Autodesk Inventor part; units mm, degrees
ref_plane "YZ Plane" through (0, 0, 0) normal (1, 0, 0) x (0, 1, 0)
ref_plane "XZ Plane" through (0, 0, 0) normal (0, 1, 0) x (-1, 0, 0)
ref_plane "XY Plane" through (0, 0, 0) normal (0, 0, 1) x (1, 0, 0)
sketch "Sketch1" plane through (0, 0, 0) normal (0, 1, 0) x (-1, 0, 0)
  circle A0 centre (0, 0) radius 40.5
  circle A1 centre (0, 0) radius 61
  dimension "d0" = 81
  dimension "d1" = 122
extrude "Extrusion1" add sketch "Sketch1" along normal blind 24
sketch "Sketch2" plane through (0, 24, 0) normal (0, 1, 0) x (1, 0, 0)
  circle A0 centre (0, 0) radius 51 construction
  point P0 (-51, 0)
  point P1 (25.5, -44.1673)
  point P2 (25.5, 44.1673)
  dimension "d4" = 102
  dimension "d7" = 360
hole "Hole1" at (-51, 24, 0) at (25.5, 24, 44.1673) at (25.5, 24, -44.1673) direction (0, -1, 0) diameter 5.5 end through all
properties part number "Adapter"
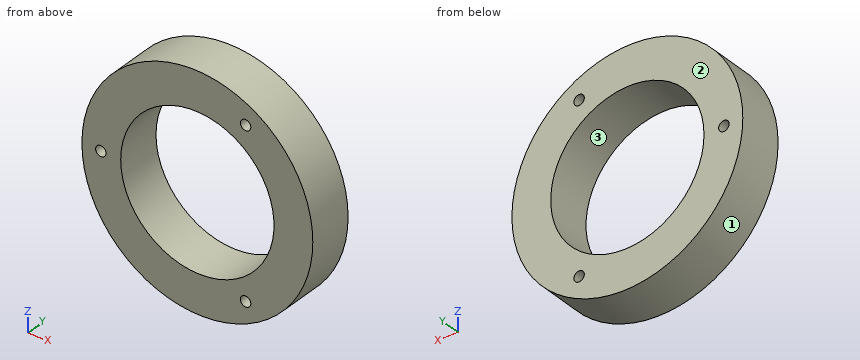
Geometry: final body of the model. Coordinates: model frame, mm. Face numbers are marked on the shaded views. Coordinates: 2 decimals unless noted, no trailing zeros. Order: outer loops, then holes, each group sorted by start corner. A loop starts at its lowest first (then second) coordinate and runs counter-clockwise, first axis right, second up.
(1) Section query D-D (y = 15). Return the cut outline in (x, z), plus the area to 3 significant figures.
(2) Material intervals for probe 1 along Z at (x, y) = (25.5, 7); probe 2 along Z at (x, y) = (27, 16.5); probe 3 along Z at (x, y) = (0, 12.75), sorted ascending.
(3) First-contact query: pin 1 (8 mm diameter, centred on x = -23, y = 6.5, fed in from +Z); pin 2 (8 mm diameter, centred on x = -39, z = -2.5, fed in from +Y); pin 3 (1.5 mm diameter, centred on y = 6, z = -31.5, fed in from -X); pin 4 (1 mm diameter, centred on x = 40.5, y = 12.5, fed in from -Z). Flat tips, straight axial feed; report the tip coordinate or a pass-through.
(4) Draft query along Z for the marked faces 1, 2 and 3. Return one class per face: pulls with the +Z half, pulls with the -Z half, needs draft (parallel to the pull), parting line crosses it, or undercut.
(5) Section query A-A (x = 0). Return the cut outline in (y, z).
(6) Section query B-B (z = 0). Return the cut outline in (x, y).
(7) Section query C-C (z = -23). Return the cut outline in (x, y).
Solution:
1. outline: circle Ø122 at (0, 0); hole circle Ø5.5 at (-51, 0); hole circle Ø81 at (0, 0); hole circle Ø5.5 at (25.5, -44.17); hole circle Ø5.5 at (25.5, 44.17)
1. area: 6,470 mm2
2. probe 1: z = -55.41 to -46.92, -41.42 to -31.46, 31.46 to 41.42, 46.92 to 55.41
2. probe 2: z = -54.7 to -46.47, -41.86 to -30.19, 30.19 to 41.86, 46.47 to 54.7
2. probe 3: z = -61 to -40.5, 40.5 to 61
3. pin 1: stops at z = 57.97
3. pin 2: stops at y = 24
3. pin 3: stops at x = -52.68
3. pin 4: stops at z = -46.05
4. face 1: parting line crosses it
4. face 2: needs draft
4. face 3: undercut
5. outline: (0, -61) - (24, -61) - (24, -40.5) - (0, -40.5) - close; (0, 40.5) - (24, 40.5) - (24, 61) - (0, 61) - close
6. outline: (-61, 0) - (-53.75, 0) - (-53.75, 24) - (-61, 24) - close; (-48.25, 0) - (-40.5, 0) - (-40.5, 24) - (-48.25, 24) - close; (40.5, 0) - (61, 0) - (61, 24) - (40.5, 24) - close
7. outline: (-56.5, 0) - (-33.34, 0) - (-33.34, 24) - (-56.5, 24) - close; (33.34, 0) - (56.5, 0) - (56.5, 24) - (33.34, 24) - close
